Autodesk Inventor part; units mm, degrees
ref_plane "YZ Plane" through (0, 0, 0) normal (1, 0, 0) x (0, 1, 0)
ref_plane "XZ Plane" through (0, 0, 0) normal (0, 1, 0) x (-1, 0, 0)
ref_plane "XY Plane" through (0, 0, 0) normal (0, 0, 1) x (1, 0, 0)
sketch "Sketch1" plane through (0, 0, 0) normal (0, 1, 0) x (-1, 0, 0)
  line L0 (18, -21) -> (-18, -21)
  line L1 (-21, -18) -> (-21, 18)
  line L2 (-18, 21) -> (18, 21)
  line L3 (21, 18) -> (21, -18)
  line L4 (21, -21) -> (-21, 21) construction
  line L5 (-21, -21) -> (21, 21) construction
  line L6 (21, 18) -> (18, 21)
  line L7 (-21, -18) -> (-18, -21)
  line L8 (-18, 21) -> (-21, 18)
  line L9 (21, -18) -> (18, -21)
  line L10 (19.5, 19.5) -> (15.0999, 15.0999) construction
  circle A0 centre (15.5563, 15.5563) radius 1.75
  circle A1 centre (-15.5563, 15.5563) radius 1.75
  circle A2 centre (-15.5563, -15.5563) radius 1.75
  circle A3 centre (15.5563, -15.5563) radius 1.75
  circle A4 centre (0, 0) radius 6.75
  line L11 (-15.5563, 15.5563) -> (15.5563, -15.5563) construction
  dimension "d0" = 42
  dimension "d1" = 42
  dimension "d2" = 3
  dimension "d3" = 3
  dimension "d4" = 3
  dimension "d5" = 3
  dimension "d6" = 3
  dimension "d7" = 3
  dimension "d8" = 3
  dimension "d9" = 3
  dimension "d11" = 3.5
  dimension "d14" = 360
  dimension "d16" = 13.5
  dimension "d20" = 22
extrude "Extrusion1" add sketch "Sketch1" along normal blind 1
sketch "Sketch3" plane through (0, 0, 0) normal (0, -1, 0) x (1, 0, 0)
  circle A0 centre (0, 0) radius 6.75
  circle A1 centre (-15.5563, 15.5563) radius 1.75
  line L0 (-21, 18) -> (-18, 21)
  line L1 (-21, -18) -> (-21, 18)
  line L2 (-18, -21) -> (-21, -18)
  line L3 (18, -21) -> (-18, -21)
  line L4 (21, -18) -> (18, -21)
  line L5 (21, 18) -> (21, -18)
  line L6 (18, 21) -> (21, 18)
  line L7 (-18, 21) -> (18, 21)
  circle A2 centre (-15.5563, 15.5563) radius 4
  circle A3 centre (-15.5563, -15.5563) radius 4
  circle A4 centre (15.5563, -15.5563) radius 4
  circle A5 centre (15.5563, 15.5563) radius 4
  dimension "d28" = 8
  dimension "d31" = 360
extrude "Extrusion3" add sketch "Sketch3" along normal blind 1 contours L0 L7 L6 L5 L4 L3 L2 L1
sketch "Sketch4" plane through (0, -1, 0) normal (0, -1, 0) x (1, 0, 0)
  circle A0 centre (0, 0) radius 6.75
  circle A1 centre (15.5563, 15.5563) radius 4
  circle A2 centre (15.5563, -15.5563) radius 4
  line L0 (-18, -21) -> (18, -21)
  line L1 (18, -21) -> (21, -18)
  line L2 (21, -18) -> (21, 18)
  line L3 (21, 18) -> (18, 21)
  line L4 (18, 21) -> (-18, 21)
  line L5 (-9.5, 6.75) -> (-9.5, 21)
  line L6 (-11.5, -6.75) -> (-11.5, -21)
  line L7 (-11.5, -6.75) -> (0, -6.75)
  line L8 (-9.5, 6.75) -> (0, 6.75)
  line L9 (0, 0) -> (0, 21) construction
  line L10 (0, 0) -> (0, -21) construction
  line L11 (0, 0) -> (21, 0) construction
  line L12 (21, 18) -> (21, -18) construction
  line L13 (0, 0) -> (-21, 0) construction
  line L14 (-21, -18) -> (-21, 18) construction
  circle A3 centre (0, 0) radius 6.75 construction
  dimension "d39" = 32.5
  dimension "d40" = 30.5
  dimension "d103" = 13.5
extrude "Extrusion4" add sketch "Sketch4" along normal blind 20 contours A0 L8 L5 L4 L3 L2 L1 L0 L6 L7
chamfer "Chamfer1" distance 2 angle 45 1 edges at (-11.5, -11, -6.75)
sketch "Sketch5" plane through (-18, 1, 21) normal (0, 0, 1) x (1, 0, 0)
  line L0 (0, 0) -> (36, 0)
  circle A0 centre (11.7, -12) radius 1
  line L1 (6.5, -2) -> (6.5, -22)
  point P0 (18, -1)
  dimension "d46" = 2
  dimension "d47" = 12
  dimension "d108" = 5.2
extrude "Extrusion5" cut sketch "Sketch5" against normal blind 20
sketch "Sketch6" plane through (18, 1, -21) normal (0, 0, -1) x (-1, 0, 0)
  line L0 (0, 0) -> (36, 0)
  circle A0 centre (24.3, -12) radius 2.5
  line L1 (29.5, -2) -> (29.5, -22)
  line L2 (29.5, -22) -> (0, -22)
  point P0 (18, -1)
  dimension "d51" = 5
  dimension "d52" = 12
  dimension "d72" = 10
  dimension "d107" = 5.2
extrude "Extrusion6" cut sketch "Sketch6" against normal blind 6
sketch "Sketch7" plane through (0, -21, -6.75) normal (0, 0, 1) x (1, 0, 0)
  line L0 (-9.5, 0) -> (-9.5, 20)
  circle A0 centre (-6.3, 10) radius 3.2
  line L1 (-18, 22) -> (18, 22)
  line L2 (-11.5, 20) -> (-11.5, 0)
  point P0 (0, 21)
  dimension "d57" = 12
  dimension "d109" = 5.2
sketch "Sketch8" plane through (-6.3, -11, -15) normal (0, 0, -1) x (-1, 0, 0)
  circle A0 centre (0, 0) radius 2.5
  circle A1 centre (0, 0) radius 1
  line L0 (5.2, 10) -> (5.2, -10)
  line L1 (-6.3, 10) -> (3.2, 10)
  point P0 (-6.3, 11)
  dimension "d56" = 2
  dimension "d104" = 5.2
  dimension "d105" = 10
  dimension "d106" = 5
loft "Loft1" cut profiles "Sketch8", "Sketch7" contours A1 / all
sketch "Sketch9" plane through (0, -21, 0) normal (0, -1, 0) x (1, 0, 0)
  line L0 (-11.5, -8.75) -> (-11.5, -21)
  line L1 (-11.5, -21) -> (18, -21)
  line L2 (-10.5, -17.4) -> (-2.1, -17.4)
  line L3 (-2.1, -17.4) -> (-2.1, -20)
  line L4 (-2.1, -20) -> (-10.5, -20)
  line L5 (-10.5, -20) -> (-10.5, -17.4)
  dimension "d73" = 8.4
  dimension "d74" = 2.6
  dimension "d75" = 1
  dimension "d76" = 1
extrude "Extrusion8" cut sketch "Sketch9" against normal blind 16
sketch "Sketch12" plane through (0, -21, 0) normal (0, -1, 0) x (1, 0, 0)
  line L0 (-10.5, -17.4) -> (-2.1, -17.4)
  line L1 (-2.1, -17.4) -> (-2.1, -15.6)
  line L2 (-2.1, -15.6) -> (-10.5, -15.6)
  line L3 (-10.5, -15.6) -> (-10.5, -17.4)
  line L4 (-2.1, -20) -> (-10.5, -20)
  dimension "d79" = 1.8
extrude "Extrusion9" cut sketch "Sketch12" against normal blind 4.5
sketch "Sketch21" plane through (18, 1, -21) normal (0, 0, -1) x (-1, 0, 0)
  circle A0 centre (24.3, -12) radius 2.5
  line L0 (0, 0) -> (36, 0)
  line L1 (29.5, -2) -> (29.5, -22)
  line L2 (29.5, -12) -> (29.5, 0)
  line L3 (29.5, 0) -> (19.1, 0)
  line L4 (19.1, 0) -> (19.1, -12)
  arc A1 (19.1, -12) -> (29.5, -12) centre (24.3, -12) ccw
  point P0 (29.5, -23)
  point P1 (18, -1)
extrude "Extrusion14" add sketch "Sketch21" along normal blind 5
sketch "Sketch23" plane through (-9.5, -1, 6.75) normal (-1, 0, 0) x (0, 0, 1)
  arc A0 (10.315, -5.15) -> (10.305, -2.15) centre (10.31, -3.65) ccw
  line L0 (14.25, 0) -> (14.25, -20)
  arc A1 (4.305, -2.17) -> (4.315, -5.17) centre (4.31, -3.67) ccw
  line L1 (11.25, 0) -> (-24.75, 0)
  line L2 (10.305, -2.15) -> (4.305, -2.17)
  line L3 (4.315, -5.17) -> (10.315, -5.15)
  arc A2 (10.31, -17.85) -> (10.31, -14.85) centre (10.31, -16.35) ccw
  arc A3 (4.31, -14.85) -> (4.31, -17.85) centre (4.31, -16.35) ccw
  line L4 (14.25, -20) -> (0, -20)
  line L5 (10.31, -14.85) -> (4.31, -14.85)
  line L6 (4.31, -17.85) -> (10.31, -17.85)
  point P0 (-6.75, 1)
  dimension "d110" = 3
  dimension "d111" = 3.94
  dimension "d112" = 3
  dimension "d113" = 9.94
  dimension "d114" = 3.65
  dimension "d115" = 3.67
  dimension "d116" = 3
  dimension "d117" = 3
  dimension "d118" = 3.94
  dimension "d119" = 9.94
  dimension "d120" = 3.65
  dimension "d121" = 3.65
extrude "Extrusion15" cut sketch "Sketch23" against normal blind 30.5
sketch "Sketch24" plane through (0, -21, 0) normal (0, -1, 0) x (1, 0, 0)
  line L0 (9, 21) -> (9, 9)
  line L1 (-9.5, 11.06) -> (21, 11.06)
  line L2 (9, 9) -> (21, 9)
  line L3 (21, -18) -> (21, 18)
  line L4 (18, 21) -> (-9.5, 21)
  line L5 (9, 21) -> (18, 21)
  line L6 (21, 18) -> (21, 9)
  line L7 (18, 21) -> (21, 18)
  line L8 (21, 18) -> (18, 21)
  point P0 (0, 0)
  dimension "d124" = 12
  dimension "d125" = 12
extrude "Extrusion16" cut sketch "Sketch24" against normal blind 20
equation "\"d3\" = d2"
equation "\"d5\" = d4"
equation "\"d7\" = d6"
equation "\"d9\" = d8"
Geometry check sheet. Reference: the model listing, model coordinates, mm. A direction names the side the tool comes from. Round coordinates to 2 decimals unless told otherwise and drop trailing zeros. Order: outer loops, then holes, each group sorted by start corner. A loop starts at its lowest first (then second) coordinate and runs counter-clockwise, first axis right, second up. Notation, with made-up numbers: (71.25, -32) - (86.25, -32) arc R18 cw to (86.25, -21) - close; hole circle Ø9 at (26.5, 64). An arc over 180 degrees is marked (long way). Use a Markdown table: item, result. Add a question column.
(1) Release check for a two-part mould opening along Y. For faces 1 (the cylindrical face through (-0.38, -4.68, 18.56)), 2 (the flat face through (-9.5, -11, 14)), 3 (the flat face through (13.8, 0, -16.4)), 4 (the flat face through (-7, -12, -15)) record: pulls with the +Y half, pulls with the -Y half, needs draft (parallel to the pull), parting line crosses it, or undercut.
(2) Material ranges on line 1 along Y through (x, z) = (4, 14); line 2 along Z through (x, y) = (-1, -8.75); line 3 along Z through (x, y) = (-2.5, -5.25), recorded low to high. Write a range as [from, to].
(3) Tool access check on faces 5 (the cylindrical face through (-7.45, -13.22, -16.22)), 6 (the flat face through (-6, -16.5, -16)), 7 (the flat face through (-5, -11, 6.75)). Record the directions out of +Z, -Z, +X, -X, +Y, -Y that give a thin tool (end or side, any length) a straight path to the whole face; none if there is none.
(4) Sectioned sample at D-D, the plane y = -7. Enter the section's corners in (x, z).
(5) Depth check by flat-ended pin: pin 1 (5 mm diameter, centred on x = 4, y = -18, fed in from -Z); pin 2 (0.9 mm diameter, centred on y = -18.5, z = -16.5, fed in from -X); pin 3 (9 mm diameter, centred on x = 16, z = 16, fed in from -Y); pin 4 (1.2 mm diameter, centred on x = -6.3, y = -11, fed in from -Z). Enter the tip coordinate at first touch or a pass-through.
(6) Sectioned sample at B-B, the plane x = 16.5. Enter the section's corners in (y, z).
(7) Sectioned sample at C-C, the plane z = -10.5. Enter the section's corners in (x, y).
(8) Sectioned sample at A-A, the plane y = -17.35. Enter the section's corners in (x, z).
Answers below:
| question | item | result |
|---|---|---|
| 1 | face 1 | undercut |
| 1 | face 2 | needs draft |
| 1 | face 3 | pulls with the -Y half |
| 1 | face 4 | undercut |
| 2 | line 1 | [-21, -18.85], [-15.85, -6.16], [-3.16, 1] |
| 2 | line 2 | [-21, -6.75], [6.75, 21] |
| 2 | line 3 | [-26, -20], [-17.4, -6.75], [6.75, 9.68], [18.43, 21] |
| 3 | face 5 | -Z |
| 3 | face 6 | -Y |
| 3 | face 7 | -X, -Y |
| 4 | outline | (-11.5, -26) - (-1.1, -26) - (-1.1, -21) - (18, -21) - (21, -18) - (21, 9) - (9, 9) - (9, 21) - (-9.5, 21) - (-9.5, 6.75) - (0, 6.75) arc R6.75 cw to (0, -6.75) - (-9.5, -6.75) - (-11.5, -8.75) - close; hole (-10.5, -20) - (-2.1, -20) - (-2.1, -17.4) - (-10.5, -17.4) - close; hole circle Ø8 at (15.56, -15.56) |
| 5 | pin 1 | z = -21 |
| 5 | pin 2 | x = -11.5 |
| 5 | pin 3 | y = -1 |
| 5 | pin 4 | through |
| 6 | outline | (-21, -21) - (1, -21) - (1, -17.03) - (0, -17.03) - (0, -19.44) - (-21, -19.44) - close; (-21, -11.67) - (0, -11.67) - (0, -14.08) - (1, -14.08) - (1, 14.08) - (0, 14.08) - (0, 11.67) - (-1, 11.67) - (-1, 9) - (-21, 9) - close; (-1, 19.44) - (0, 19.44) - (0, 17.03) - (1, 17.03) - (1, 21) - (-1, 21) - close |
| 7 | outline | (-21, -1) - (-11.5, -1) - (-11.5, -21) - (21, -21) - (21, 1) - (-21, 1) - close; hole circle Ø4.4 at (-6.3, -11) |
| 8 | outline | (-11.5, -21) - (18, -21) - (21, -18) - (21, 9) - (9, 9) - (9, 9.56) - (-9.5, 9.56) - (-9.5, 6.75) - (0, 6.75) arc R6.75 cw to (0, -6.75) - (-9.5, -6.75) - (-11.5, -8.75) - close; (-9.5, 18.56) - (9, 18.56) - (9, 21) - (-9.5, 21) - close; hole (-10.5, -20) - (-2.1, -20) - (-2.1, -15.6) - (-10.5, -15.6) - close; hole circle Ø8 at (15.56, -15.56) |
